Can you work these out from the model? Positions are in its coordinate system, mm. A direction names the side the tool comes from. Round coordinates to 2 decimals unless told otherwise and drop trailing zeros. Loops run counter-clockwise (first coordinate to the right, second up) from the corner with the lowest first, then second, coordinate; pieces in that order, holes last. Notation, with made-up numbers: (71.5, 61.5) -> (130.5, 61.5) arc R35 cw to (130.5, 100.5) -> close; hole circle Ø4 at (12, 53.5). An arc over 180 degrees is marked (long way). Use a Markdown table: item, result.
from build123d import *

# Parameters (mm, degrees)
SKETCH1_W           = 26.246666667
SKETCH1_H           = 70
SKETCH1_R           = 2.15
BOSS_EXTRUDE1_DEPTH = 4.45
FILLET1_R           = 3


with BuildPart() as part:
    # Sketch1 → Boss-Extrude1 (new body)
    with BuildSketch(Plane(origin=(7.062589735, 0, -4.077588085), x_dir=(0.5, 0, 0.866025404), z_dir=(-0.866025404, 0, 0.5))):
        Polygon((14.47543448, 209.798849573), (14.47543448, 136.798849573), (6.702101147, 118.055853922), (56.49543448, 118.055853922), (48.722101147, 136.798849573), (48.722101147, 209.798849573), align=None)
        with Locations((31.598767814, 171.798849573)):
            Rectangle(SKETCH1_W, SKETCH1_H, mode=Mode.SUBTRACT)
        with Locations((51.49543448, 122.055853922)):
            Circle(SKETCH1_R, mode=Mode.SUBTRACT)
        with Locations((44.722101147, 132.798849573)):
            Circle(SKETCH1_R, mode=Mode.SUBTRACT)
        with Locations((11.702101147, 122.055853922)):
            Circle(SKETCH1_R, mode=Mode.SUBTRACT)
        with Locations((18.47543448, 132.798849573)):
            Circle(SKETCH1_R, mode=Mode.SUBTRACT)
        Polygon((45.924572578, 122.055853922), (17.27296305, 122.055853922), (23.47543448, 132.798849573), (39.722101147, 132.798849573), align=None, mode=Mode.SUBTRACT)
    extrude(amount=-BOSS_EXTRUDE1_DEPTH)

    # Fillet1
    fillet1_edges = [part.edges().sort_by_distance(p)[0] for p in [
        (12.340546832, 118.055853922, 0.614101768),
        (37.237213499, 118.055853922, 43.736393373),
        (33.350546832, 209.798849573, 37.004489235),
        (16.227213499, 209.798849573, 7.346005906),
    ]]
    fillet(fillet1_edges, radius=FILLET1_R)


solid = part.part
1. If we mould it in two halves opening along Z, with no side actions, what happens to faces 1 (the flat face through (33.596, 157.346, 32.979)), 2 (the cylindrical face through (31.18, 134.93, 33.31)), 3 (the flat face through (25, 209.799, 22))? For each: +Z half, -Z half, draft (parallel to the pull), parting line (faces both ways), or undercut.
Answer sheet:
| item | result |
|---|---|
| face 1 | -Z half |
| face 2 | undercut |
| face 3 | draft |
2. I need wall thicknesses on line 1 (Y direction, x = 29.75, z = 32.5); line 2 (Y direction, x = 17, z = 10); line 3 (Z direction, x = 34, y = 202.5). Which ranges of each line are inside material? Lowest first, please.
Answer sheet:
| item | result |
|---|---|
| line 1 | y = 118.06 to 122.06, 127.09 to 131.48, 134.11 to 136.8, 206.8 to 209.8 |
| line 2 | y = 118.06 to 131.1, 134.5 to 209.78 |
| line 3 | z = 33.68 to 36.63 |
3. Will these pins go through, and if not, where does the flat tip stop? pin 1 Ø8 at (y, z) = (187, 31) entering from +X; pin 2 Ø1.5 at (x, y) = (17.5, 193) entering from -Z.
Answer sheet:
| item | result |
|---|---|
| pin 1 | stops at x = 34.76 |
| pin 2 | stops at z = 6.23 |
4. I want a section at C-C (y = 128.5). Please give me the cut outline in (x, z), plus the area to 3 significant figures.
Answer sheet:
| item | result |
|---|---|
| outline | (12.58, 5.48) -> (16.43, 3.25) -> (21.41, 11.88) -> (17.56, 14.1) -> close; (28.16, 32.47) -> (32.02, 30.25) -> (37, 38.87) -> (33.14, 41.1) -> close |
| area | 88.6 mm² |
5. I want a section at B-B (z = 21). Please give me the cut outline in (x, y), plus the area to 3 significant figures.
Answer sheet:
| item | result |
|---|---|
| outline | (21.54, 118.06) -> (26.68, 118.06) -> (26.68, 122.06) -> (21.54, 122.06) -> close; (21.54, 132.8) -> (26.68, 132.8) -> (26.68, 136.8) -> (21.54, 136.8) -> close; (21.54, 206.8) -> (26.68, 206.8) -> (26.68, 209.8) -> (21.54, 209.8) -> close |
| area | 56.5 mm² |
6. Which directions (+Z, -Z, +X, -X, +Y, -Y) give clear straight access to the entire face, cutting with the end or side of a thin tool? Please do faces 4 (the flat face through (31.32, 171.31, 33.56)), 5 (the flat face through (33.32, 171.31, 37.02)), 6 (the flat face through (18.2, 171.309, 10.826)), 7 (the cylindrical face through (16.682, 208.897, 8.071)).
Answer sheet:
| item | result |
|---|---|
| face 4 | -Z, -X |
| face 5 | +Z, +X, +Y |
| face 6 | +Z, +X |
| face 7 | -Z, -X, +Y |
7. I want a section at A-A (y = 158.5). Please give me the cut outline in (x, z), plus the area to 3 significant figures.
Answer sheet:
| item | result |
|---|---|
| outline | (14.3, 8.46) -> (18.15, 6.23) -> (20.15, 9.7) -> (16.3, 11.92) -> close; (29.42, 34.65) -> (33.28, 32.43) -> (35.28, 35.89) -> (31.42, 38.12) -> close |
| area | 35.6 mm² |
